Source: CAD feature listing. Evaluate the final solid. Frame: model axes, mm. Face numbers are marked on the shaded views. A direction names the side the tool comes from. Give positions to 0.01 mm unless a question says otherwise; leave off trailing zeros. Order: outer loops, then holes, each group sorted by start corner. A loop starts at its lowest first (then second) coordinate and runs counter-clockwise, first axis right, second up. Notation, with made-up numbers: M 23,25 L 72,25 A29 ccw 72,61 Z; hole C 5,49 d5. An arc over 180 degrees is marked long. Answer as a JSON object with one key per item and string values. Group by question number.
1. Section query A-A (x = 10). Output: boundary loops of the cut face in (y, z), plus the area to 3 significant figures.
2. Section query C-C (y = 19). Output: boundary loops of the cut face in (x, z), plus the area to 3 significant figures.
3. Material intervals for L1, parallel to Z at x = 3, y = 18; L2, parallel to Z at x = 6, y = 21.5; L3, parallel to X at y = 12, z = -2.25, sorted ascending. Write a range as [from, to].
4. Section query D-D (z = 8). Output: boundary loops of the cut face in (x, y), plus the area to 3 significant figures.
5. Set-up query: the marked faces 1 and 2. Return all of +Z, -Z, +X, -X, +Y, -Y with unobstructed straight access to the full face (end or side cutting, diameter ignored); none if empty.
6. Pull-direction query (X, two-part tool) for the marked faces 3, 4 and 5; classes: +X half, -X half, draft (parallel to the pull), parting line (faces both ways), or undercut.
7. Pin query (flat end, axial travel): P1, Ø1.5, axis at x = 20.5, z = 1, coming from the +Y side; P2, Ø8.5, axis at y = 19, z = 0, coming from the +X side; P3, Ø6, axis at x = 18.5, z = 0, coming from the -Y side. Return the tip coordinate at first contact, or that it passes through.
8. Section query B-B (z = 0). Count the separate pieces of the cut face and the enclosed holes in it, plus the area to 3 significant figures.
from build123d import *

# Parameters (mm, degrees)
SKETCH1_W               = 30
SKETCH1_H               = 30
BOSS_EXTRUDE1_DEPTH     = 10
CUT_EXTRUDE3_DEPTH      = 10
CUT_EXTRUDE3_DEPTH_BACK = 10
SKETCH7_OUTSIDE_W       = 41.38
SKETCH7_OUTSIDE_H       = 41.38
CUT_EXTRUDE4_DEPTH      = 7.5
BOSS_EXTRUDE3_REACH     = 50.089
BOSS_EXTRUDE3_START     = 4.5
DIAMETER_HOLE1_D        = 5.3
BOSS_EXTRUDE4_DEPTH     = 1
BOSS_EXTRUDE5_DEPTH     = 1
DIAMETER_HOLE2_D        = 5.3
DIAMETER_HOLE3_D        = 5.3


with BuildPart() as part:
    # Sketch1 → Boss-Extrude1 (new, symmetric)
    with BuildSketch(Plane.XY):
        with Locations((15, 15)):
            Rectangle(SKETCH1_W, SKETCH1_H)
    extrude(amount=BOSS_EXTRUDE1_DEPTH, both=True)

    # Sketch7 outside → Cut-Extrude3 (cut, two sides: drawn at the far end of the back side and taken through both)
    with BuildSketch(Plane.XY.offset(-CUT_EXTRUDE3_DEPTH_BACK)):
        with Locations((15, 15)):
            Rectangle(SKETCH7_OUTSIDE_W, SKETCH7_OUTSIDE_H)
        with BuildLine():
            Line((0, 0), (30, 0))
            Line((30, 0), (30, 4.085786438))
            ThreePointArc((30, 4.085786438), (29.923879533, 4.46846987), (29.707106781, 4.792893219))
            Line((29.707106781, 4.792893219), (4.792893219, 29.707106781))
            ThreePointArc((4.792893219, 29.707106781), (4.46846987, 29.923879533), (4.085786438, 30))
            Line((4.085786438, 30), (0, 30))
            Line((0, 30), (0, 0))
        make_face(mode=Mode.SUBTRACT)
    extrude(amount=CUT_EXTRUDE3_DEPTH + CUT_EXTRUDE3_DEPTH_BACK, mode=Mode.SUBTRACT)

    # Sketch8 → Cut-Extrude4 (cut, symmetric)
    with BuildSketch(Plane.XY):
        Polygon((3.163601628, 30), (4.5, 4.5), (30, 4.5), (30, 30), align=None)
    extrude(amount=CUT_EXTRUDE4_DEPTH, both=True, mode=Mode.SUBTRACT)

    # Boss-Extrude3: up to this plane
    boss_extrude3_end = Plane(origin=(3.163601628, 30, -7.5), z_dir=(-0.9986295347545743, -0.05233595624293714, 0))
    # Sketch9 → Boss-Extrude3 (add, up to the surface)
    with BuildSketch(Plane(origin=(0, 0, 0), x_dir=(0, 0, -1), z_dir=(1, 0, 0)).offset(BOSS_EXTRUDE3_START), mode=Mode.PRIVATE) as boss_extrude3_sk1:
        with BuildLine():
            Line((4.468669433, 18.530088202), (5.421224791, 10.5))
            Line((5.421224791, 10.5), (-5.421224791, 10.5))
            Line((-5.421224791, 10.5), (-4.468669433, 18.530088202))
            ThreePointArc((-4.468669433, 18.530088202), (0, 22.5), (4.468669433, 18.530088202))
        make_face()
    boss_extrude3_tool1 = split(extrude(boss_extrude3_sk1.sketch, amount=-BOSS_EXTRUDE3_REACH, mode=Mode.PRIVATE), bisect_by=boss_extrude3_end, keep=Keep.BOTH, mode=Mode.PRIVATE)
    add(boss_extrude3_tool1.solids().sort_by_distance((4.5, 15.863056, 0))[0])

    # Diameter Hole1 (through all)
    with Locations(Plane(origin=(0, 30, 0), x_dir=(1, 0, 0), z_dir=(0, 1, 0))):
        with Locations((18, 0)):
            Hole(DIAMETER_HOLE1_D / 2)

    # Sketch12 → Boss-Extrude4 (add)
    with BuildSketch(Plane(origin=(0, 0, 0), x_dir=(0, 0, -1), z_dir=(1, 0, 0))):
        with BuildLine():
            Line((2.7, 24), (-2.7, 24))
            ThreePointArc((-2.7, 24), (-2.912132034, 23.912132034), (-3, 23.7))
            Line((-3, 23.7), (-3, 21.3))
            ThreePointArc((-3, 21.3), (-2.912132034, 21.087867966), (-2.7, 21))
            Line((-2.7, 21), (2.7, 21))
            ThreePointArc((2.7, 21), (2.912132034, 21.087867966), (3, 21.3))
            Line((3, 21.3), (3, 23.7))
            ThreePointArc((3, 23.7), (2.912132034, 23.912132034), (2.7, 24))
        make_face()
        with BuildLine():
            Line((2.7, 11), (-2.7, 11))
            ThreePointArc((-2.7, 11), (-2.912132034, 10.912132034), (-3, 10.7))
            Line((-3, 10.7), (-3, 5.3))
            ThreePointArc((-3, 5.3), (-2.912132034, 5.087867966), (-2.7, 5))
            Line((-2.7, 5), (2.7, 5))
            ThreePointArc((2.7, 5), (2.912132034, 5.087867966), (3, 5.3))
            Line((3, 5.3), (3, 10.7))
            ThreePointArc((3, 10.7), (2.912132034, 10.912132034), (2.7, 11))
        make_face()
    extrude(amount=-BOSS_EXTRUDE4_DEPTH)

    # Sketch13 → Boss-Extrude5 (add)
    with BuildSketch(Plane(origin=(0, 0, 0), x_dir=(1, 0, 0), z_dir=(0, 1, 0))):
        with BuildLine():
            Line((10.5, -3), (12.7, -3))
            ThreePointArc((12.7, -3), (12.912132034, -2.912132034), (13, -2.7))
            Line((13, -2.7), (13, -0.5))
            Line((13, -0.5), (10.5, -0.5))
            Line((10.5, -0.5), (10.5, -3))
        make_face()
        with BuildLine():
            Line((7.3, -3), (9.5, -3))
            Line((9.5, -3), (9.5, -0.5))
            Line((9.5, -0.5), (7, -0.5))
            Line((7, -0.5), (7, -2.7))
            ThreePointArc((7, -2.7), (7.087867966, -2.912132034), (7.3, -3))
        make_face()
        with BuildLine():
            Line((7.3, 3), (9.5, 3))
            Line((9.5, 3), (9.5, 0.5))
            Line((9.5, 0.5), (7, 0.5))
            Line((7, 0.5), (7, 2.7))
            ThreePointArc((7, 2.7), (7.087867966, 2.912132034), (7.3, 3))
        make_face()
        with BuildLine():
            Line((10.5, 3), (12.7, 3))
            ThreePointArc((12.7, 3), (12.912132034, 2.912132034), (13, 2.7))
            Line((13, 2.7), (13, 0.5))
            Line((13, 0.5), (10.5, 0.5))
            Line((10.5, 0.5), (10.5, 3))
        make_face()
    extrude(amount=-BOSS_EXTRUDE5_DEPTH)

    # Diameter Hole2 (through all)
    with Locations(Plane(origin=(30, 10, 0), x_dir=(0, 1, 0), z_dir=(1, 0, 0))):
        with Locations((8, 0)):
            Hole(DIAMETER_HOLE2_D / 2)

    # Diameter Hole3 (through all)
    with Locations(Plane(origin=(0, 30, 0), x_dir=(1, 0, 0), z_dir=(0, 1, 0))):
        with Locations((10, 0)):
            Hole(DIAMETER_HOLE3_D / 2)


solid = part.part
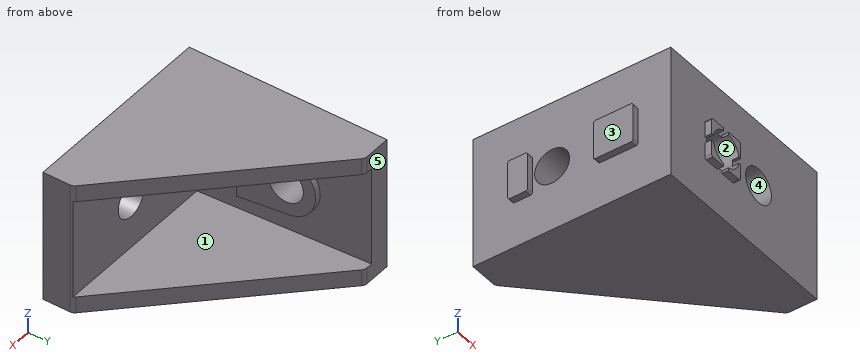
Answer sheet:
{
 "1": {"outline": "M 0,-10 L 24.5,-10 L 24.5,-7.5 L 4.5,-7.5 L 4.5,-2.65 L 0,-2.65 Z; M 0,2.65 L 4.5,2.65 L 4.5,7.5 L 24.5,7.5 L 24.5,10 L 0,10 Z", "area": "166 mm^2"},
 "2": {"outline": "M 0,-10 L 15.5,-10 L 15.5,-7.5 L 3.74,-7.5 L 3.74,-4.39 L 4.5,-4.39 L 4.5,-2.45 L 0,-2.45 Z; M 0,2.45 L 4.5,2.45 L 4.5,4.39 L 3.74,4.39 L 3.74,7.5 L 15.5,7.5 L 15.5,10 L 0,10 Z", "area": "118 mm^2"},
 "3": {"L1": "[-10, -2.65], [2.65, 10]", "L2": "[-10, -7.5], [7.5, 10]", "L3": "[0, 4.5]"},
 "4": {"outline": "M 0,0 L 30,0 L 30,4.09 A1 ccw 29.71,4.79 L 4.79,29.71 A1 ccw 4.09,30 L 0,30 Z", "area": "575 mm^2"},
 "5": {"face 1": "+X, +Y", "face 2": "+Y, -Y"},
 "6": {"face 3": "-X half", "face 4": "undercut", "face 5": "draft"},
 "7": {"P1": "y = 4.5", "P2": "x = 4.5", "P3": "y = 0"},
 "8": {"separate pieces": "4", "enclosed holes": "0", "area": "178 mm^2"}
}
